Can you work these out from the model? Positions are in its coordinate system, mm. A direction names the side the tool comes from. Give positions to 0.01 mm unless a question says otherwise; leave off trailing zeros. Order: outer loops, then holes, each group sorted by start corner. A loop starts at its lowest first (then second) coordinate and runs counter-clockwise, first axis right, second up.
Item 1: I'm going to push flat-ended pins straight in: pin 1 Ø2.5 at (x, z) = (78.5, -21) entering from +Y; pin 2 Ø1.2 at (y, z) = (4.5, -13.5) entering from +X; pin 3 Ø5 at (x, z) = (78.5, 21) entering from +Y; pin 4 Ø1.2 at (y, z) = (4.5, -4) entering from -X. Where does each tip first touch, or does it pass through?
Item 2: If we mould it in two halves opening along Z, with no side actions, what happens to faces 1 (the flat face through (-79, 3.5, 0)), 2 (the cylindrical face through (-76.592, 1.774, -21.601)), 3 (the flat face through (-1, 3, -27.5))? For each: +Z half, -Z half, draft (parallel to the pull), parting line (faces both ways), or undercut.
Item 3: I want a section at A-A, the plane x = 78.5. Write out the boundary of the cut face in (y, z), then the cut area to 4 significant figures.
Item 4: Which directions (+Z, -Z, +X, -X, +Y, -Y) give clear straight access to the entire face, cutting with the end or side of a thin tool? Please do faces 4 (the flat face through (78, 3.5, 0)), 5 (the flat face through (-1, 6, 0)).
Item 5: If I drill on line 1 along X through (y, z) = (1.7, -21); line 2 along Z through (x, y) = (-78.5, 1.9); line 3 along X through (y, z) = (3, -20.5), over which ranges is the centre line in solid material (lowest first)?
Item 6: I want a section at B-B, the plane z = 21. Write out the boundary of the cut face in (x, y), then the cut area to 3 significant figures.
Item 7: I want a section at C-C, the plane z = 9. Write out the boundary of the cut face in (x, y).
```python
from build123d import *

# Parameters (mm, degrees)
ESQUISSE1_W             = 172
ESQUISSE1_H             = 55
BOSS_EXTRU_1_DEPTH      = 3.5
ESQUISSE2_R             = 2
ENL_V_MAT_EXTRU_1_DEPTH = 6
ESQUISSE3_W             = 142
ESQUISSE3_H             = 55
BOSS_EXTRU_2_DEPTH      = 2.5


with BuildPart() as part:
    # Esquisse1 → Boss.-Extru.1 (new body)
    with BuildSketch(Plane(origin=(0, 0, 0), x_dir=(1, 0, 0), z_dir=(0, 1, 0))):
        Rectangle(ESQUISSE1_W, ESQUISSE1_H)
    extrude(amount=BOSS_EXTRU_1_DEPTH)

    # Esquisse2 → Enlèv. mat.-Extru.1 (cut)
    with BuildSketch(Plane(origin=(0, 3.5, 0), x_dir=(1, 0, 0), z_dir=(0, 1, 0))):
        with Locations((-78.5, 21)):
            Circle(ESQUISSE2_R)
        with Locations((-78.5, -21)):
            Circle(ESQUISSE2_R)
        with Locations((78.5, -21)):
            Circle(ESQUISSE2_R)
        with Locations((78.5, 21)):
            Circle(ESQUISSE2_R)
    extrude(amount=-ENL_V_MAT_EXTRU_1_DEPTH, mode=Mode.SUBTRACT)

    # Esquisse3 → Boss.-Extru.2 (add)
    with BuildSketch(Plane(origin=(0, 3.5, 0), x_dir=(1, 0, 0), z_dir=(0, 1, 0))):
        Rectangle(ESQUISSE3_W, ESQUISSE3_H)
    extrude(amount=BOSS_EXTRU_2_DEPTH)


solid = part.part
```
Results list:
1. pin 1: passes through
1. pin 2: stops at x = 71
1. pin 3: stops at y = 3.5
1. pin 4: stops at x = -71
2. face 1: draft
2. face 2: undercut
2. face 3: -Z half
3. outline: (0, -27.5) - (3.5, -27.5) - (3.5, -23) - (0, -23) - close; (0, -19) - (3.5, -19) - (3.5, 19) - (0, 19) - close; (0, 23) - (3.5, 23) - (3.5, 27.5) - (0, 27.5) - close
3. area: 164.5 mm2
4. face 4: +Z, -Z, +X, +Y
4. face 5: +Z, -Z, +X, -X, +Y
5. line 1: x = -86 to -80.5, -76.5 to 76.5, 80.5 to 86
5. line 2: z = -27.5 to -23, -19 to 19, 23 to 27.5
5. line 3: x = -86 to -80.44, -76.56 to 76.56, 80.44 to 86
6. outline: (-86, 0) - (-80.5, 0) - (-80.5, 3.5) - (-86, 3.5) - close; (-76.5, 0) - (76.5, 0) - (76.5, 3.5) - (71, 3.5) - (71, 6) - (-71, 6) - (-71, 3.5) - (-76.5, 3.5) - close; (80.5, 0) - (86, 0) - (86, 3.5) - (80.5, 3.5) - close
6. area: 929 mm2
7. outline: (-86, 0) - (86, 0) - (86, 3.5) - (71, 3.5) - (71, 6) - (-71, 6) - (-71, 3.5) - (-86, 3.5) - close
